```python
from build123d import *

# Parameters (mm, degrees)
SKETCH1_W                       = 38.1
SKETCH1_H                       = 30.48
EXTRUDE1_DEPTH                  = 6.35
SKETCH2_W                       = 38.1
SKETCH2_H                       = 6.35
EXTRUDE2_DEPTH                  = 22.86
F_16_0_177_DIAMETER_HOLE3_D     = 4.4958
F_16_0_177_DIAMETER_HOLE3_DEPTH = 58.42
F_16_0_177_DIAMETER_HOLE3_TIP   = 1.350674586
SKETCH6_R                       = 15.875
CUT_EXTRUDE2_DEPTH              = 25.4
F_10_32_TAPPED_HOLE1_D          = 4.0386
CIRPATTERN1_COUNT               = 2
CIRPATTERN1_ANGLE               = 45


with BuildPart() as part:
    # Sketch1 → Extrude1 (new body)
    with BuildSketch(Plane(origin=(0, 0, 0), x_dir=(1, 0, 0), z_dir=(0, 1, 0))):
        with Locations((0, -2.54)):
            Rectangle(SKETCH1_W, SKETCH1_H)
    extrude(amount=EXTRUDE1_DEPTH)

    # Sketch2 → Extrude2 (add)
    with BuildSketch(Plane(origin=(0, 6.35, 0), x_dir=(-1, 0, 0), z_dir=(0, 1, 0))):
        with Locations((0, 14.605)):
            Rectangle(SKETCH2_W, SKETCH2_H)
    extrude(amount=EXTRUDE2_DEPTH)

    # #16 (0.177) Diameter Hole3
    with Locations(Plane(origin=(0, 6.35, 6.35), x_dir=(0, 0, 1), z_dir=(0, 1, 0))):
        with Locations((0, 0), (-12.7, 0)):
            Hole(F_16_0_177_DIAMETER_HOLE3_D / 2, depth=F_16_0_177_DIAMETER_HOLE3_DEPTH)
            with Locations((0, 0, -(F_16_0_177_DIAMETER_HOLE3_DEPTH + F_16_0_177_DIAMETER_HOLE3_TIP / 2))):  # 118° drill point
                Cone(0, F_16_0_177_DIAMETER_HOLE3_D / 2, F_16_0_177_DIAMETER_HOLE3_TIP, mode=Mode.SUBTRACT)

    # Sketch6 → Cut-Extrude2 (cut)
    with BuildSketch(Plane.XY.offset(17.78)):
        with Locations((0, 29.21)):
            Circle(SKETCH6_R)
    extrude(amount=-CUT_EXTRUDE2_DEPTH, mode=Mode.SUBTRACT)

    # #10-32 Tapped Hole1 (through all)
    with Locations(Plane(origin=(7.776127346, 10.436767899, 17.78), x_dir=(1, 0, 0), z_dir=(0, 0, 1))):
        with Locations((0, 0)):
            f_10_32_tapped_hole1 = Hole(F_10_32_TAPPED_HOLE1_D / 2)

    # CirPattern1: #10-32 Tapped Hole1 ×2 about axis
    cirpattern1_axis = Axis((0, 29.21, 35.207153655), (0, 0, -1))
    for i in range(1, CIRPATTERN1_COUNT):
        add(f_10_32_tapped_hole1.rotate(cirpattern1_axis, i * CIRPATTERN1_ANGLE / (CIRPATTERN1_COUNT - 1)), mode=Mode.SUBTRACT)


solid = part.part
```
The listing builds one solid part. Answer for the finished solid, in the listing's coordinates (mm). A direction names the side the tool comes from. Give positions to 0.01 mm unless a question says otherwise; leave off trailing zeros. Order: outer loops, then holes, each group sorted by start corner. A loop starts at its lowest first (then second) coordinate and runs counter-clockwise, first axis right, second up. Notation, with made-up numbers: M -39,67.5 L -15,67.5 A10 cw -15,84.5 Z; hole C -28,66.5 d9. An arc over 180 degrees is marked long. Put each result on its own line as item: value. Start each with the question number.
Item 1: Which of the six approach directions +Z, -Z, +X, -X, +Y, -Y give full straight-line access (tool end or side, diameter ignored) to faces 5 (the face through (0, 6.35, -1)), 6 (the face through (-19.05, 5, 9))?
Item 2: For a pull along Z with two mould halves and no side action, classify faces 1 (the face through (0, 11, 17.78)), 2 (the face through (0.675, 3.131, -8.494)), 3 (the face through (19.05, 5, 9)), 4 (the face through (0, 13, 11.43)) as +Z half, -Z half, draft (parallel to the pull), parting line (faces both ways), or undercut.
Item 3: Flat-ended cylindrical pins translate along their axes: P1, Ø3, axis at x = -7.78, y = 10.44, coming from the -Z side; P2, Ø4, axis at x = 2, z = -5, coming from the +Y side. Find the tip coordinate at first contact, or state that the pin passes through.
Item 4: The part is cut by section D-D, the plane y = 2.5. Determine the outline of the cut face in (x, z), and give its area (3 significant figures).
Item 5: The part is cut by section B-B, the plane x = 0. Determine the outline of the cut face in (y, z) (3 decimals), and give its area (3 significant figures).
Item 6: The part is cut by section A-A, the plane z = 6.35. Determine the outline of the cut face in (x, y).
Item 7: Find the intervals of material crossed by line 1 along X through (y, z) = (5, 6.35); line 2 along Y through (x, z) = (11, 4.5); line 3 along Z through (x, y) = (4, 9.5), in increasing order.
Item 8: The part is cut by section C-C, the plane y = 21.75. Determine the outline of the cut face in (x, z).
Answer key:
1. face 5: -Z, +X, -X, +Y
1. face 6: +Z, -Z, -X, +Y, -Y
2. face 1: +Z half
2. face 2: undercut
2. face 3: draft
2. face 4: -Z half
3. P1: passes through
3. P2: stops at y = 6.35
4. outline: M -19.05,-12.7 L 19.05,-12.7 L 19.05,17.78 L -19.05,17.78 Z; hole C 0,-6.35 d4.5; hole C 0,6.35 d4.5
4. area: 1,130 mm²
5. outline: M 0,-12.7 L 6.35,-12.7 L 6.35,-8.598 L 0,-8.598 Z; M 0,-4.102 L 6.35,-4.102 L 6.35,4.102 L 0,4.102 Z; M 0,8.598 L 6.35,8.598 L 6.35,11.43 L 13.335,11.43 L 13.335,17.78 L 0,17.78 Z
5. area: 181 mm²
6. outline: M -19.05,0 L -2.25,0 L -2.25,6.35 L -19.05,6.35 Z; M 2.25,0 L 19.05,0 L 19.05,6.35 L 2.25,6.35 Z
7. line 1: x = -19.05 to -2.25, 2.25 to 19.05
7. line 2: y = 0 to 6.35
7. line 3: z = 11.43 to 17.78
8. outline: M -19.05,11.43 L -14.01,11.43 L -14.01,17.78 L -19.05,17.78 Z; M 14.01,11.43 L 19.05,11.43 L 19.05,17.78 L 14.01,17.78 Z
